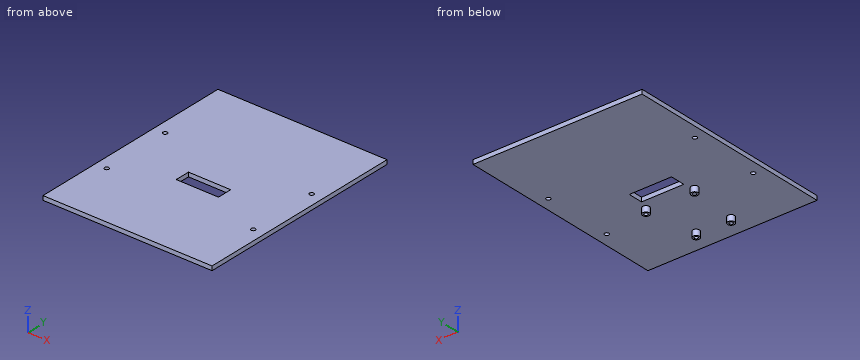
from build123d import *

# Parameters (mm, degrees)
SKETCH1_W           = 120
SKETCH1_H           = 150
SKETCH1_R           = 1.5
BOSS_EXTRUDE1_DEPTH = 3
SKETCH2_R           = 2.403365395
SKETCH2_R_2         = 1.25
SKETCH2_R_3         = 2.397656746
BOSS_EXTRUDE2_DEPTH = 4
SKETCH3_W           = 30
SKETCH3_H           = 10.5
CUT_EXTRUDE1_DEPTH  = 10


with BuildPart() as part:
    # Sketch1 → Boss-Extrude1 (new body)
    with BuildSketch(Plane.XY):
        with Locations((60, 75)):
            Rectangle(SKETCH1_W, SKETCH1_H)
        with Locations((112, 95)):
            Circle(SKETCH1_R, mode=Mode.SUBTRACT)
        with Locations((112, 45)):
            Circle(SKETCH1_R, mode=Mode.SUBTRACT)
        with Locations(Location((8, 45, 0), (0, 0, 180))):
            Circle(SKETCH1_R, mode=Mode.SUBTRACT)
        with Locations(Location((8, 95, 0), (0, 0, 180))):
            Circle(SKETCH1_R, mode=Mode.SUBTRACT)
    extrude(amount=BOSS_EXTRUDE1_DEPTH)

    # Sketch2 → Boss-Extrude2 (add)
    # profile 1 of 4: a face of its own
    with BuildSketch(Plane(origin=(0, 0, 0), x_dir=(-1, 0, 0), z_dir=(0, 0, -1))):
        with Locations(Location((-42.75, 53.304125965, 0), (0, 0, 180))):
            Circle(SKETCH2_R)
        with Locations(Location((-42.75, 53.304125965, 0), (0, 0, 180))):
            Circle(SKETCH2_R_2, mode=Mode.SUBTRACT)
    # profile 2 of 4: a face of its own
    with BuildSketch(Plane(origin=(0, 0, 0), x_dir=(-1, 0, 0), z_dir=(0, 0, -1))):
        with Locations(Location((-47.6, 16.154125965, 0), (0, 0, 180))):
            Circle(SKETCH2_R_3)
        with Locations(Location((-47.6, 16.154125965, 0), (0, 0, 180))):
            Circle(SKETCH2_R_2, mode=Mode.SUBTRACT)
    # profile 3 of 4: a face of its own
    with BuildSketch(Plane(origin=(0, 0, 0), x_dir=(-1, 0, 0), z_dir=(0, 0, -1))):
        with Locations((-72.4, 16.154125965)):
            Circle(SKETCH2_R_3)
        with Locations((-72.4, 16.154125965)):
            Circle(SKETCH2_R_2, mode=Mode.SUBTRACT)
    # profile 4 of 4: a face of its own
    with BuildSketch(Plane(origin=(0, 0, 0), x_dir=(-1, 0, 0), z_dir=(0, 0, -1))):
        with Locations((-77.25, 53.304125965)):
            Circle(SKETCH2_R)
        with Locations((-77.25, 53.304125965)):
            Circle(SKETCH2_R_2, mode=Mode.SUBTRACT)
    extrude(amount=BOSS_EXTRUDE2_DEPTH)

    # Sketch3 → Cut-Extrude1 (cut)
    with BuildSketch(Plane(origin=(0, 0, 0), x_dir=(-1, 0, 0), z_dir=(0, 0, -1))):
        with Locations((-60, 65.111028977)):
            Rectangle(SKETCH3_W, SKETCH3_H)
    extrude(amount=-CUT_EXTRUDE1_DEPTH, mode=Mode.SUBTRACT)


solid = part.part
Here's how the part is built. I have some questions about the finished solid (model axes, mm). Round coordinates to 2 decimals unless told otherwise and drop trailing zeros. Loops run counter-clockwise (first coordinate to the right, second up) from the corner with the lowest first, then second, coordinate; pieces in that order, holes last.
1. If we section it at B-B on y = 66.5: Write out the boundary of the cut face in (x, z), plus the area to 3 significant figures.
Answer list:
outline: (0, 0) - (45, 0) - (45, 3) - (0, 3) - close; (75, 0) - (120, 0) - (120, 3) - (75, 3) - close
area: 270 mm2
2. For P1, Ø2, axis at x = 77.5, y = 54, coming from the -Z side; P2, Ø0.8, axis at x = 42.5, y = 53.5, coming from the -Z side; P3, Ø2.5, axis at x = 8, y = 95, coming from the -Z side, each with a flat end and sliding along its axis, tell me the tip position at first contact or that it passes through.
Answer list:
P1: stops at z = -4
P2: stops at z = 0
P3: passes through
3. If we section it at A-A on z = 1.5: Write out the boundary of the cut face in (x, y), plus the area to 3 significant figures.
Answer list:
outline: (0, 0) - (120, 0) - (120, 150) - (0, 150) - close; hole circle Ø3 at (8, 45); hole circle Ø3 at (8, 95); hole (45, 59.86) - (75, 59.86) - (75, 70.36) - (45, 70.36) - close; hole circle Ø3 at (112, 45); hole circle Ø3 at (112, 95)
area: 17,700 mm2
4. If I drill on line 1 along Y through (x, z) = (8, 2.2); line 2 along X through (y, z) = (95, 1.3); line 3 along X through (y, z) = (62, 2), over which ranges is the centre line in solid material (lowest first)?
Answer list:
line 1: y = 0 to 43.5, 46.5 to 93.5, 96.5 to 150
line 2: x = 0 to 6.5, 9.5 to 110.5, 113.5 to 120
line 3: x = 0 to 45, 75 to 120
5. If we section it at C-C on x = 95: Write out the boundary of the cut face in (y, z).
Answer list:
outline: (0, 0) - (150, 0) - (150, 3) - (0, 3) - close
